Part model, mm, in its own coordinate system. Face numbers are marked on the shaded views. A direction names the side the tool comes from. Coordinates: 2 decimals unless noted, no trailing zeros. Order: outer loops, then holes, each group sorted by start corner. A loop starts at its lowest first (then second) coordinate and runs counter-clockwise, first axis right, second up. Notation, with made-up numbers: M 0,65 L 53,65 A25 cw 53,84 Z; hole C 66,85.5 d4. An arc over 180 degrees is marked long. Answer in a Markdown table with one row per item. Add a question column.
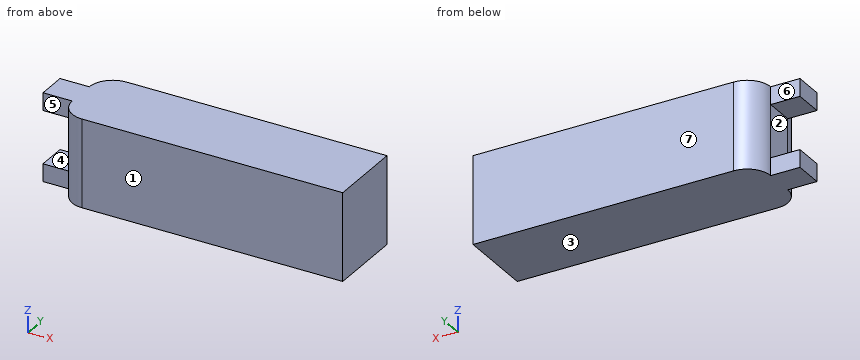
from build123d import *

# Parameters (mm, degrees)
SKETCH1_W           = 97
SKETCH1_H           = 30
BOSS_EXTRUDE1_DEPTH = 26
FILLET1_R           = 8
SKETCH2_W           = 6
SKETCH2_H           = 10
BOSS_EXTRUDE2_DEPTH = 10


with BuildPart() as part:
    # Sketch1 → Boss-Extrude1 (new body)
    with BuildSketch(Plane(origin=(0, 0, 0), x_dir=(1, 0, 0), z_dir=(0, 1, 0))):
        with Locations((48.5, 15)):
            Rectangle(SKETCH1_W, SKETCH1_H)
    extrude(amount=BOSS_EXTRUDE1_DEPTH)

    # Fillet1
    fillet1_edges = [part.edges().sort_by_distance(p)[0] for p in [
        (0, 26, -15),
        (0, 0, -15),
    ]]
    fillet(fillet1_edges, radius=FILLET1_R)

    # Sketch2 → Boss-Extrude2 (add)
    with BuildSketch(Plane.ZY):
        with Locations((-27, 13)):
            Rectangle(SKETCH2_W, SKETCH2_H)
        with Locations((-3, 13)):
            Rectangle(SKETCH2_W, SKETCH2_H)
    extrude(amount=BOSS_EXTRUDE2_DEPTH)


solid = part.part
(1) Slice it at D-D (y = 4.5). List the corners of the cut face in (x, z), and give its area (3 significant figures).
(2) Drop flat-ended pins along their axis: P1, Ø4, axis at y = 3, z = -23, coming from the -X side; P2, Ø6, axis at y = 12.5, z = -10, coming from the -X side; P3, Ø1.8, axis at x = -7, z = -27.5, coming from the -Y side. Give the stop position or say it passes through.
(3) 3-axis set-ups, long thin cutter, end or side, ignore diameter. For the marked faces 4, 5, 6 and 7: which of +Z, -Z, +X, -X, +Y, -Y reach the whole face in a straight line?
(4) Slice it at B-B (z = -9.5). List the corners of the cut face in (x, y).
(5) Slice it at A-A (y = 14.75). List the corners of the cut face in (x, z), and give its area (3 significant figures).
(6) Pull direction Z, two halves, no side cores. Call the marked faces 1, 2 and 3: pulls with the +Z half, pulls with the -Z half, needs draft (parallel to the pull), parting line crosses it, or undercut.
(7) Slice it at C-C (z = -3). List the corners of the cut face in (x, y).
(8) Wall check: line 1 (X direction, y = 9.25, z = -18.5); line 2 (X direction, y = 20.25, z = -15.75); line 3 (Y direction, x = 2.5, z = -15). Give the ranges that are in metal, low to high.
Computed:
| question | item | result |
|---|---|---|
| 1 | outline | M 0.81,-30 L 97,-30 L 97,0 L 0.81,0 Z |
| 1 | area | 2,890 mm^2 |
| 2 | P1 | stops at x = 0.58 |
| 2 | P2 | stops at x = 0 |
| 2 | P3 | stops at y = 8 |
| 3 | face 4 | -X, +Y, -Y |
| 3 | face 5 | +Z, -Z, -X, -Y |
| 3 | face 6 | +Z, -Z, -X, +Y |
| 3 | face 7 | +Z, -Z, +X, -X, +Y |
| 4 | outline | M 0,8 A8 ccw 8,0 L 97,0 L 97,26 L 8,26 A8 ccw 0,18 Z |
| 5 | outline | M -10,-30 L 97,-30 L 97,0 L -10,0 L -10,-6 L 0,-6 L 0,-24 L -10,-24 Z |
| 5 | area | 3,030 mm^2 |
| 6 | face 1 | needs draft |
| 6 | face 2 | undercut |
| 6 | face 3 | pulls with the -Z half |
| 7 | outline | M -10,8 L 0,8 A8 ccw 8,0 L 97,0 L 97,26 L 8,26 A8 ccw 0,18 L -10,18 Z |
| 8 | line 1 | x = 0 to 97 |
| 8 | line 2 | x = 0.32 to 97 |
| 8 | line 3 | y = 2.19 to 23.81 |
